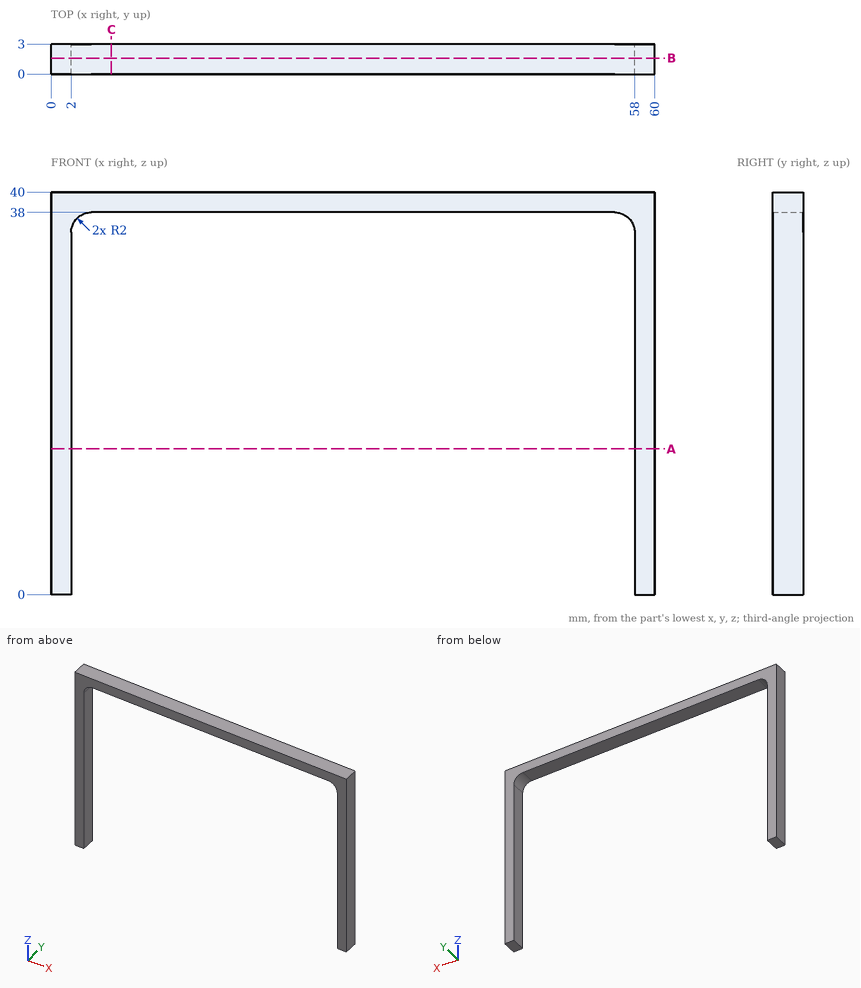
Here's the drawing with two shaded views (mm, measured from the low corner). I have some questions. Round coordinates to 2 decimals unless told otherwise and drop trailing zeros. Write each loop counter-clockwise with the first axis right and the second up, starting at its lowest first coordinate (ties: lowest second). Pieces come first, ordered by that corner, then holes. Notation, with made-up numbers: M -14,50.25 L 19,50.25 A23 cw 19,78.25 Z; hole C 70,-10 d3. An arc over 180 degrees is marked long. Write each question's results on one line, items separated by ' | '. Start each with the question number.
1. I need wall thicknesses on L1, parallel to X at y = 1, z = 7; L2, parallel to Z at x = 50.5, y = 2.25; L3, parallel to X at y = 2.3, z = 37. Which ranges of each line are inside material? Lowest first, please. Write a range as from..to.
2. Imagine slicing it at B-B on y = 1.6. List the corners of the cut face in (x, z) for me, and give its area (3 significant figures).
3. Imagine slicing it at C-C on x = 6. List the corners of the cut face in (y, z) for me.
4. Imagine slicing it at A-A on z = 14.5. List the corners of the cut face in (x, y) for me, and give its area (3 significant figures).
Result sheet:
1) L1: x = 0..2, 58..60 | L2: z = 38..40 | L3: x = 0..2.27, 57.73..60
2) outline: M 0,0 L 2,0 L 2,36 A2 cw 4,38 L 56,38 A2 cw 58,36 L 58,0 L 60,0 L 60,40 L 0,40 Z | area: 274 mm^2
3) outline: M 0,38 L 3,38 L 3,40 L 0,40 Z
4) outline: M 0,0 L 2,0 L 2,3 L 0,3 Z; M 58,0 L 60,0 L 60,3 L 58,3 Z | area: 12.0 mm^2
